```python
from build123d import *

# Parameters (mm, degrees)
SKETCH2_W                    = 32
SKETCH2_H                    = 15
BOSS_EXTRUDE1_DEPTH          = 6.35
TAP_DRILL_FOR_M8X1_25_TAP1_D = 6.8
FILLET1_R                    = 7.5


with BuildPart() as part:
    # Sketch2 → Boss-Extrude1 (new body)
    with BuildSketch(Plane(origin=(0, 0, 0), x_dir=(1, 0, 0), z_dir=(0, 1, 0))):
        with Locations((16, 7.5)):
            Rectangle(SKETCH2_W, SKETCH2_H)
    extrude(amount=BOSS_EXTRUDE1_DEPTH)

    # Tap Drill for M8x1.25 Tap1 (through all)
    with Locations(Plane(origin=(8, 6.35, -7.5), x_dir=(0, 0, 1), z_dir=(0, 1, 0))):
        with Locations((0, 0), (0, 16)):
            Hole(TAP_DRILL_FOR_M8X1_25_TAP1_D / 2)

    # Fillet1
    fillet1_edges = [part.edges().sort_by_distance(p)[0] for p in [
        (32, 3.175, 0),
        (32, 3.175, -15),
        (0, 3.175, -15),
        (0, 3.175, 0),
    ]]
    fillet(fillet1_edges, radius=FILLET1_R - 0.0001)  # a hair under: the kernel refuses the full size


solid = part.part
```
Design review of the part built by this model. Coordinates are the model's own, in mm. Round coordinates to 2 decimals unless told otherwise and drop trailing zeros. Write each loop counter-clockwise with the first axis right and the second up, starting at its lowest first coordinate (ties: lowest second). Pieces come first, ordered by that corner, then holes.
Item 1: We need section B-B on y = 1.5. State how many separate pieces and enclosed holes the cut face has, and give its area (3 significant figures).
Item 2: Clearance check with flat-ended pins moving along their axes: pin 1 Ø4 at (x, z) = (24, -7.5) entering from -Y; pin 2 Ø1.5 at (y, z) = (3, -12.5) entering from +X; pin 3 Ø1.5 at (y, z) = (4.5, -1.5) entering from +X. State where each tip first meets the part, or that it passes through.
Item 3: We need section A-A on x = 24. Write out the cut boundary in (y, z), and give its area (3 significant figures).
Item 4: The part is to be moulded in two halves that separate along Z. For faces 1 (the flat face through (16, 3, -15)), 2 (the flat face through (16, 0, -8)), 3 (the cylindrical face through (25.021, 3.131, -10.743)), say which applies: +Z half, -Z half, draft (parallel to the pull), parting line (faces both ways), or undercut.
Item 5: We need section D-D on z = -6.75. Write out the cut boundary in (x, y).
Item 6: We need section C-C on z = -10.25. Write out the cut boundary in (x, y).
Item 7: For probe 1 along X at (y, z) = (3.75, -7.5); probe 2 along X at (y, z) = (2.5, -9.5); probe 3 along Z at (x, y) = (10, 4), list the stretches that pass through material, from the lowest coordinate up.
Returned:
1. separate pieces: 1
1. enclosed holes: 2
1. area: 359 mm2
2. pin 1: passes through
2. pin 2: stops at x = 30.68
2. pin 3: stops at x = 29.86
3. outline: (0, -15) - (6.35, -15) - (6.35, -10.9) - (0, -10.9) - close; (0, -4.1) - (6.35, -4.1) - (6.35, 0) - (0, 0) - close
3. area: 52.1 mm2
4. face 1: -Z half
4. face 2: draft
4. face 3: undercut
5. outline: (0.04, 0) - (4.68, 0) - (4.68, 6.35) - (0.04, 6.35) - close; (11.32, 0) - (20.68, 0) - (20.68, 6.35) - (11.32, 6.35) - close; (27.32, 0) - (31.96, 0) - (31.96, 6.35) - (27.32, 6.35) - close
6. outline: (0.52, 0) - (6, 0) - (6, 6.35) - (0.52, 6.35) - close; (10, 0) - (22, 0) - (22, 6.35) - (10, 6.35) - close; (26, 0) - (31.48, 0) - (31.48, 6.35) - (26, 6.35) - close
7. probe 1: x = 0 to 4.6, 11.4 to 20.6, 27.4 to 32
7. probe 2: x = 0.27 to 5.25, 10.75 to 21.25, 26.75 to 31.73
7. probe 3: z = -15 to -10.25, -4.75 to 0
